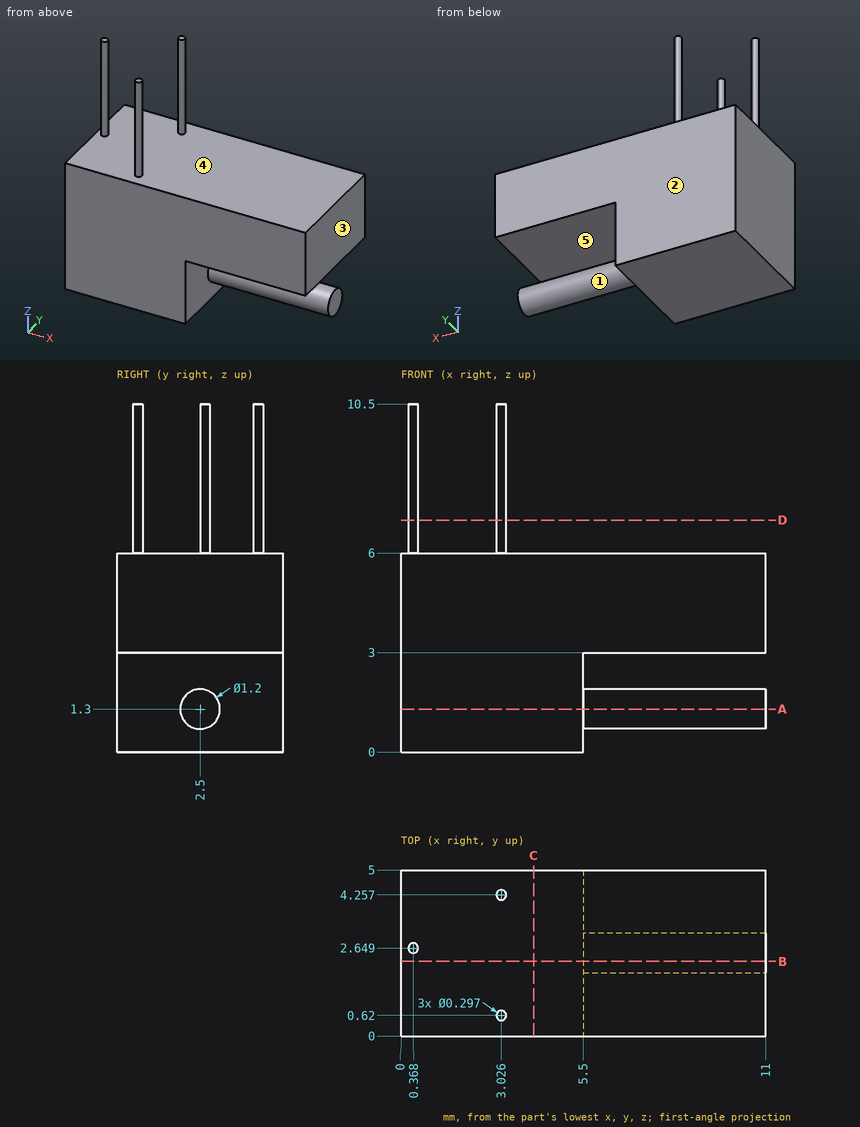
Drawing for the job (mm, zero at the part's lowest x, y, z). A direction names the side the tool comes from. Give positions to 0.01 mm unless a question says otherwise; leave off trailing zeros. Loops run counter-clockwise (first coordinate to the right, second up) from the corner with the lowest first, then second, coordinate; pieces in that order, holes last.
(1) Pin check, flat tip, straight feed: pin 1 (1.5 mm diameter, centred on x = 9, y = 4, fed in from +Z). Stop position of the tip, or through.
Return value:
pin 1: stops at z = 6
(2) Band-saw the part on D-D (z = 7). Write the cut outline in (x, y) (1 decimal).
Return value:
outline: circle Ø0.3 at (0.4, 2.6); circle Ø0.3 at (3, 0.6); circle Ø0.3 at (3, 4.3)
(3) Band-saw the part on A-A (z = 1.3). Write the cut outline in (x, y).
Return value:
outline: (0, 0) - (5.5, 0) - (5.5, 1.9) - (11, 1.9) - (11, 3.1) - (5.5, 3.1) - (5.5, 5) - (0, 5) - close
(4) Drill centre lines: line 1 along Z through (x, y) = (6.25, 2.5); line 2 along Z through (x, y) = (1.75, 4.65); line 3 along Z through (x, y) = (7.75, 1.8). Where is each one in solid material? Low to high.
Return value:
line 1: z = 0.7 to 1.9, 3 to 6
line 2: z = 0 to 6
line 3: z = 3 to 6
(5) 3-axis set-ups, long thin cutter, end or side, ignore diameter. For the marked faces 1 and 2: which of +Z, -Z, +X, -X, +Y, -Y reach the whole face in a straight line?
Return value:
face 1: +X
face 2: +Z, -Z, +X, -X, +Y
(6) Band-saw the part on C-C (x = 4). Write the cut outline in (y, z), and give its area (3 significant figures).
Return value:
outline: (0, 0) - (5, 0) - (5, 6) - (0, 6) - close
area: 30.0 mm2
(7) Pull direction Z, two halves, no side cores. Call the marked faces 3, 4 and 5: pulls with the +Z half, pulls with the -Z half, needs draft (parallel to the pull), parting line crosses it, or undercut.
Return value:
face 3: needs draft
face 4: pulls with the +Z half
face 5: undercut
(8) Band-saw the part on B-B (y = 2.25). Write the cut outline in (x, z) (1 decimal), and give its area (3 significant figures).
Return value:
outline: (0, 0) - (5.5, 0) - (5.5, 0.8) - (11, 0.8) - (11, 1.8) - (5.5, 1.8) - (5.5, 3) - (11, 3) - (11, 6) - (0, 6) - close
area: 55.5 mm2
